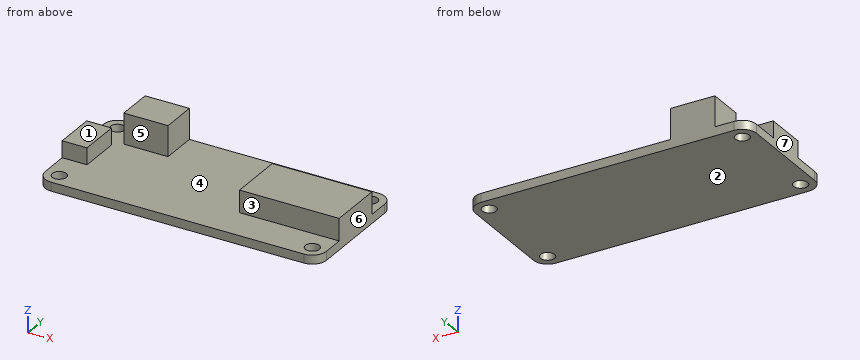
from build123d import *

# Parameters (mm, degrees)
F0_R     = 1.27
F1_DEPTH = 1.6
F2_W     = 4.5
F2_H     = 7.5
F3_DEPTH = 3
F4_W     = 18
F4_H     = 10
F5_DEPTH = 4
F6_W     = 8
F6_H     = 6.5
F7_DEPTH = 5.5


with BuildPart() as f1:
    # F0 (on Top) → F1 (new body)
    with BuildSketch(Plane.XY):
        with BuildLine():
            ThreePointArc((25.4, 8.89), (24.656051, 10.686051), (22.86, 11.43))
            Line((22.86, 11.43), (-22.86, 11.43))
            ThreePointArc((-22.86, 11.43), (-24.656051, 10.686051), (-25.4, 8.89))
            Line((-25.4, 8.89), (-25.4, -8.89))
            ThreePointArc((-25.4, -8.89), (-24.656051, -10.686051), (-22.86, -11.43))
            Line((-22.86, -11.43), (22.86, -11.43))
            ThreePointArc((22.86, -11.43), (24.656051, -10.686051), (25.4, -8.89))
            Line((25.4, -8.89), (25.4, 8.89))
        make_face()
        with Locations((-22.86, -8.89)):
            Circle(F0_R, mode=Mode.SUBTRACT)
        with Locations((22.86, -8.89)):
            Circle(F0_R, mode=Mode.SUBTRACT)
        with Locations((-22.86, 8.89)):
            Circle(F0_R, mode=Mode.SUBTRACT)
        with Locations((22.86, 8.89)):
            Circle(F0_R, mode=Mode.SUBTRACT)
    extrude(amount=F1_DEPTH)

    # F2 (on face) → F3 (join)
    with BuildSketch(Plane.XY.offset(1.6)):
        with Locations((-23.15, 0)):
            Rectangle(F2_W, F2_H)
    extrude(amount=F3_DEPTH)

    # F4 (on face) → F5 (join)
    with BuildSketch(Plane.XY.offset(1.6)):
        with Locations((16.4, 0)):
            Rectangle(F4_W, F4_H)
    extrude(amount=F5_DEPTH)

    # F6 (on face) → F7 (join)
    with BuildSketch(Plane.XY.offset(1.6)):
        with Locations((-15.4, 8.18)):
            Rectangle(F6_W, F6_H)
    extrude(amount=F7_DEPTH)


solid = f1.part
Build history of the part. All positions in model axes, mm. Face numbers are marked on the shaded views. A direction names the side the tool comes from. Give positions to 0.01 mm unless a question says otherwise; leave off trailing zeros. Order: outer loops, then holes, each group sorted by start corner. A loop starts at its lowest first (then second) coordinate and runs counter-clockwise, first axis right, second up. Notation, with made-up numbers: M 12,50.25 L 52,50.25 A35 ccw 52,85.25 Z; hole C 44.25,51 d9. An arc over 180 degrees is marked long. Put each result on its own line as item: value.
Item 1: Drop flat-ended pins along their axis: pin 1 Ø11.5 at (x, y) = (-4.5, -4) entering from +Z; pin 2 Ø1.6 at (y, z) = (9, 5.5) entering from +X; pin 3 Ø1.6 at (y, z) = (8.5, 5.5) entering from -X. Give the stop position or say it passes through.
Results are:
pin 1: z = 1.6
pin 2: x = -11.4
pin 3: x = -19.4
Item 2: Cut at C-C on x = -18. Write the cut outline in (y, z), then the cut area to 3 significant figures.
Results are:
outline: M -11.43,0 L 11.43,0 L 11.43,7.1 L 4.93,7.1 L 4.93,1.6 L -11.43,1.6 Z
area: 72.3 mm2
Item 3: Which spindle directions (+Z, -Z, +X, -X, +Y, -Y) get a long thin tool onto all of the face, cutting with end or side? Do the marked faces 1, 2 and 3. Say none if no direction does.
Results are:
face 1: +Z, -X, +Y, -Y
face 2: -Z, +X, -X, +Y, -Y
face 3: +Z, +X, -X, -Y
Item 4: Cut at D-D on x = 19. Write the cut outline in (y, z).
Results are:
outline: M -11.43,0 L 11.43,0 L 11.43,1.6 L 5,1.6 L 5,5.6 L -5,5.6 L -5,1.6 L -11.43,1.6 Z
Item 5: Cut at B-B on y = 3. Write the cut outline in (x, z).
Results are:
outline: M -25.4,0 L 25.4,0 L 25.4,5.6 L 7.4,5.6 L 7.4,1.6 L -20.9,1.6 L -20.9,4.6 L -25.4,4.6 Z
Item 6: Cut at A-A on z = 3. Write the cut outline in (x, y), then the cut area to 3 significant figures.
Results are:
outline: M -25.4,-3.75 L -20.9,-3.75 L -20.9,3.75 L -25.4,3.75 Z; M -19.4,4.93 L -11.4,4.93 L -11.4,11.43 L -19.4,11.43 Z; M 7.4,-5 L 25.4,-5 L 25.4,5 L 7.4,5 Z
area: 266 mm2
Item 7: Wall check: probe 1 along Y at (x, z) = (-22.86, 1.25); probe 2 along X at (y, z) = (7.5, 3); probe 3 along Z at (x, y) = (20.5, 6). Give the ranges that are in metal, low to high.
Results are:
probe 1: -11.43 to -10.16, -7.62 to 7.62, 10.16 to 11.43
probe 2: -19.4 to -11.4
probe 3: 0 to 1.6
Item 8: Pull direction X, two halves, no side cores. Call the marked faces 4, 5, 6 and 7: +X half, -X half, draft (parallel to the pull), parting line (faces both ways), or undercut.
Results are:
face 4: undercut
face 5: draft
face 6: +X half
face 7: -X half
